The model under review builds one solid part; all positions refer to its coordinate system, in mm. Face numbers are marked on the shaded views. A direction names the side the tool comes from. Round coordinates to 2 decimals unless told otherwise and drop trailing zeros. Order: outer loops, then holes, each group sorted by start corner. A loop starts at its lowest first (then second) coordinate and runs counter-clockwise, first axis right, second up. Notation, with made-up numbers: M 35,-11 L 47,-11 A27 cw 47,8 Z; hole C 65,55.5 d6. An arc over 180 degrees is marked long. Answer as a JSON object with one key per item and string values. Group by question number.
1) Consider section C-C, the plane x = 45.5. Write out the cut boundary in (y, z), then the cut area to 3 significant figures.
2) Consider section A-A, the plane y = -22. Write out the cut boundary in (x, z), then the cut area to 3 significant figures.
3) For the marked faces 5 and 6, list the 3-axis set-ups (+Z, -Z, +X, -X, +Y, -Y) from which the entire face can be reached by the end or side of a thin tool; tool diameter is ignored.
4) Insertion check: pin 1 Ø4 at (x, z) = (10.5, 4.5) entering from -Y; pin 2 Ø0.8 at (x, z) = (46, 3.5) entering from -Y; pin 3 Ø1.6 at (x, z) = (52, 4) entering from +Y. Each pin has a flat end and moves straight along its axis. Give the tip position at first contact, or say it passes through.
5) Consider section B-B, the plane z = 6.25. Write out the cut boundary in (x, y).
6) The part is to be moulded in two halves that separate along X. For the marked faces 1, 2, 3 and 4, say which applies: +X half, -X half, draft (parallel to the pull), parting line (faces both ways), or undercut.
7) Consider section D-D, the plane x = 13.5. Write out the cut boundary in (y, z), then the cut area to 3 significant figures.
8) To check wall thickness, follow line 1 (X direction, y = -16.5, z = 2.25); line 2 (Z direction, x = 45.5, y = -37); line 3 (X direction, y = -30.5, z = 2). State the ranges of each line that lie inside material, in increasing order.
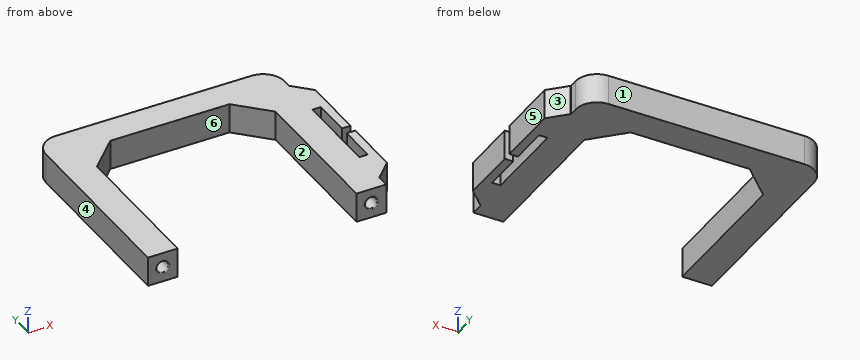
```python
from build123d import *

# Parameters (mm, degrees)
CYLINDER001_R          = 1.4
CYLINDER001_DEPTH      = 10
CYLINDER001_ROLL_ANGLE = -90
CYLINDER_R             = 1.4
CYLINDER_DEPTH         = 10
CYLINDER_ROLL_ANGLE    = -90
BOX005_W               = 2
BOX005_H               = 2
BOX005_DEPTH           = 7
BOX003_W               = 2
BOX003_H               = 20
BOX003_DEPTH           = 7
BOX001_W               = 7
BOX001_H               = 48.5
BOX001_DEPTH           = 7
BOX002_W               = 7
BOX002_H               = 48.5
BOX002_DEPTH           = 7
BOX004_W               = 4
BOX004_H               = 38.5
BOX004_DEPTH           = 7
BOX_W                  = 42
BOX_H                  = 7
BOX_DEPTH              = 7
CHAMFER_SIZE           = 3.95
CHAMFER001_SIZE        = 7
FILLET_R               = 5
FILLET001_R            = 0.25


with BuildPart() as bolt2:
    # Cylinder001 → Cylinder001 (new body)
    with BuildSketch(Plane.XY):
        Circle(CYLINDER001_R)
    extrude(amount=CYLINDER001_DEPTH)


with BuildPart() as bolt2_1:
    # Cylinder001 roll: moved
    add(bolt2.part.rotate(Axis((0, 0, 0), (1, 0, 0)), CYLINDER001_ROLL_ANGLE))


with BuildPart() as bolt2_2:
    # Cylinder001 placement: moved
    add(bolt2_1.part.moved(Location((45.5, -42, 3.5))))


with BuildPart() as bolt1:
    # Cylinder → Cylinder (new body)
    with BuildSketch(Plane.XY):
        Circle(CYLINDER_R)
    extrude(amount=CYLINDER_DEPTH)


with BuildPart() as bolt1_1:
    # Cylinder roll: moved
    add(bolt1.part.rotate(Axis((0, 0, 0), (1, 0, 0)), CYLINDER_ROLL_ANGLE))


with BuildPart() as bolt1_2:
    # Cylinder placement: moved
    add(bolt1_1.part.moved(Location((-3.5, -42, 3.5))))


with BuildPart() as cable_slot2:
    # Box005 → Box005 (new body)
    with BuildSketch(Plane(origin=(51, -21, 0), x_dir=(1, 0, 0), z_dir=(0, 0, 1))):
        with Locations((1, 1)):
            Rectangle(BOX005_W, BOX005_H)
    extrude(amount=BOX005_DEPTH)


with BuildPart() as cable_slot:
    # Box003 → Box003 (new body)
    with BuildSketch(Plane(origin=(49, -30, 0), x_dir=(1, 0, 0), z_dir=(0, 0, 1))):
        with Locations((1, 10)):
            Rectangle(BOX003_W, BOX003_H)
    extrude(amount=BOX003_DEPTH)


with BuildPart() as side1:
    # Box001 → Box001 (new body)
    with BuildSketch(Plane(origin=(-7, -41.5, 0), x_dir=(1, 0, 0), z_dir=(0, 0, 1))):
        with Locations((3.5, 24.25)):
            Rectangle(BOX001_W, BOX001_H)
    extrude(amount=BOX001_DEPTH)


with BuildPart() as side2:
    # Box002 → Box002 (new body)
    with BuildSketch(Plane(origin=(42, -41.5, 0), x_dir=(1, 0, 0), z_dir=(0, 0, 1))):
        with Locations((3.5, 24.25)):
            Rectangle(BOX002_W, BOX002_H)
    extrude(amount=BOX002_DEPTH)


with BuildPart() as cable_support:
    # Box004 → Box004 (new body)
    with BuildSketch(Plane(origin=(49, -38.5, 0), x_dir=(1, 0, 0), z_dir=(0, 0, 1))):
        with Locations((2, 19.25)):
            Rectangle(BOX004_W, BOX004_H)
    extrude(amount=BOX004_DEPTH)


with BuildPart() as holder_clamp:
    # Box → Box (new body)
    with BuildSketch(Plane.XY):
        with Locations((21, 3.5)):
            Rectangle(BOX_W, BOX_H)
    extrude(amount=BOX_DEPTH)

    # Fusion: union Side1, Side2, cable-support
    add(side1.part)
    add(side2.part)
    add(cable_support.part)

    # Cut: cut cable-slot
    add(cable_slot.part, mode=Mode.SUBTRACT)

    # Cut001: cut cable-slot2
    add(cable_slot2.part, mode=Mode.SUBTRACT)

    # Cut002: cut Bolt1
    add(bolt1_2.part, mode=Mode.SUBTRACT)

    # Cut003: cut Bolt2
    add(bolt2_2.part, mode=Mode.SUBTRACT)

    # Chamfer
    chamfer_edges = [holder_clamp.edges().sort_by_distance(p)[0] for p in [
        (53, -38.5, 3.5),
        (53, 0, 3.5),
    ]]
    chamfer(chamfer_edges, length=CHAMFER_SIZE)

    # Chamfer001
    chamfer001_edges = [holder_clamp.edges().sort_by_distance(p)[0] for p in [
        (42, 0, 3.5),
        (0, 0, 3.5),
    ]]
    chamfer(chamfer001_edges, length=CHAMFER001_SIZE)

    # Fillet
    fillet_edges = [holder_clamp.edges().sort_by_distance(p)[0] for p in [
        (49, 7, 3.5),
        (-7, 7, 3.5),
    ]]
    fillet(fillet_edges, radius=FILLET_R)

    # Fillet001
    fillet001_edges = [holder_clamp.edges().sort_by_distance(p)[0] for p in [
        (44.1, -41.5, 3.5),
        (-4.9, -41.5, 3.5),
    ]]
    fillet(fillet001_edges, radius=FILLET001_R)


solid = holder_clamp.part
```
Results list:
{
 "1": {"outline": "M -41.5,0 L 6.77,0 L 6.77,7 L -41.5,7 L -41.5,5.15 A0.25 ccw -41.25,4.9 L -32,4.9 L -32,2.1 L -41.25,2.1 A0.25 ccw -41.5,1.85 Z", "area": "311 mm^2"},
 "2": {"outline": "M -7,0 L 0,0 L 0,7 L -7,7 Z; M 42,0 L 49,0 L 49,7 L 42,7 Z; M 51,0 L 53,0 L 53,7 L 51,7 Z", "area": "112 mm^2"},
 "3": {"face 5": "+Z, -Z, +X, +Y, -Y", "face 6": "+Z, -Z, -Y"},
 "4": {"pin 1": "y = 0", "pin 2": "y = -32", "pin 3": "y = -2.15"},
 "5": {"outline": "M -7,-41.5 L 0,-41.5 L 0,-7 L 7,0 L 35,0 L 42,-7 L 42,-41.5 L 49,-41.5 L 49,-38.5 L 49.05,-38.5 L 53,-34.55 L 53,-21 L 51,-21 L 51,-30 L 49,-30 L 49,-10 L 51,-10 L 51,-19 L 53,-19 L 53,-3.95 L 49.05,0 L 49,0 L 49,2 A5 ccw 44,7 L -2,7 A5 ccw -7,2 Z"},
 "6": {"face 1": "draft", "face 2": "undercut", "face 3": "+X half", "face 4": "-X half"},
 "7": {"outline": "M 0,0 L 7,0 L 7,7 L 0,7 Z", "area": "49.0 mm^2"},
 "8": {"line 1": "-7 to 0, 42 to 49, 51 to 53", "line 2": "0 to 2.1, 4.9 to 7", "line 3": "-7 to 0, 42 to 53"}
}
